```python
from build123d import *

# Parameters (mm, degrees)
EXTRUDE_1_DEPTH     = 10
SKETCH_2_W          = 80.6
SKETCH_2_H          = 36.6
CUT_EXTRUDE_1_DEPTH = 5
SKETCH_3_W          = 73
SKETCH_3_H          = 25
CUT_EXTRUDE_2_DEPTH = 115.512008104
CUT_EXTRUDE_3_DEPTH = 3
SKETCH_5_R          = 1.6
CUT_EXTRUDE_4_DEPTH = 112.950882087


with BuildPart() as part:
    # 草图1 → 凸台-拉伸1 (new body)
    with BuildSketch(Plane.XY):
        Polygon((0, 40), (0, 63), (-8, 63), (-8, 68), (5, 68), (5, 48.19405544), (13.19405544, 40), (70.80594456, 40), (79, 48.19405544), (79, 68), (92, 68), (92, 63), (84, 63), (84, 40), (84, 0), (0, 0), align=None)
    extrude(amount=EXTRUDE_1_DEPTH)

    # 草图2 → 切除-拉伸1 (cut)
    with BuildSketch(Plane.XY.offset(10)):
        with Locations((42, 20)):
            Rectangle(SKETCH_2_W, SKETCH_2_H)
    extrude(amount=-CUT_EXTRUDE_1_DEPTH, mode=Mode.SUBTRACT)

    # 草图3 → 切除-拉伸2 (cut, through all)
    with BuildSketch(Plane.XY.offset(5)):
        with Locations((42, 20)):
            Rectangle(SKETCH_3_W, SKETCH_3_H)
    extrude(amount=-CUT_EXTRUDE_2_DEPTH, mode=Mode.SUBTRACT)

    # 草图4 → 切除-拉伸3 (cut)
    with BuildSketch(Plane.XY.offset(5)):
        Polygon((77.017311929, 30.931067044), (82.3, 27.389990557), (82.3, 13.068303431), (77.017311929, 9.448536355), align=None)
        Polygon((6.982688071, 9.448536355), (6.982688071, 30.931067044), (1.7, 27.389990557), (1.7, 13.068303431), align=None)
    extrude(amount=-CUT_EXTRUDE_3_DEPTH, mode=Mode.SUBTRACT)

    # 草图5 → 切除-拉伸4 (cut, through all)
    with BuildSketch(Plane.XZ.offset(-63)):
        with Locations(Location((87.837450425, 4.830878187, 0), (0, 0, 270))):
            Circle(SKETCH_5_R)
        with Locations(Location((-3.837450425, 4.830878187, 0), (0, 0, 90))):
            Circle(SKETCH_5_R)
    extrude(amount=-CUT_EXTRUDE_4_DEPTH, mode=Mode.SUBTRACT)


solid = part.part
```
The listing builds one solid part. Answer for the finished solid, in the listing's coordinates (mm). A direction names the side the tool comes from. Give positions to 0.01 mm unless a question says otherwise; leave off trailing zeros. Write each loop counter-clockwise with the first axis right and the second up, starting at its lowest first coordinate (ties: lowest second). Pieces come first, ordered by that corner, then holes. Notation, with made-up numbers: (30, 30) - (87, 30) arc R12 cw to (87, 42) - close; hole circle Ø1 at (48.25, 78). An arc over 180 degrees is marked (long way). Use one line per item in the form item = value. Start each with the question number.
1) Find section B-B on x = 15. Determine the outline of the cut face in (y, z).
2) Flat-ended cylindrical pins translate along their axes: pin 1 Ø2.5 at (x, z) = (88, 6) entering from -Y; pin 2 Ø3 at (y, z) = (55, 7) entering from +X; pin 3 Ø2.5 at (x, z) = (-3.84, 4.83) entering from -Y; pin 4 Ø5 at (x, z) = (87.84, 4.83) entering from +Y. Find the tip coordinate at first contact, or state that the pin passes through.
3) The mould has two halves that part along Y. Classify faces 1 (the face through (85, 68, 5)), 2 (the face through (41, 5, 5)), 3 (the face through (79, 58, 5)): pulls with the +Y half, pulls with the -Y half, needs draft (parallel to the pull), parting line crosses it, or undercut.
4) Find section C-C on y = 36. Determine the outline of the cut face in (x, z), plus the area to 3 significant figures.
5) Consider line 1 along X through (y, z) = (58.5, 8.25); line 2 along X through (y, z) = (8, 3.75); line 3 along Y through (x, z) = (27, 4.5). Determine where each line is inside the solid, lowest interval first. Write a range as from..to.
6) A tool of negligible diameter and unlimited length cuts with its end or side. For faces 4 (the face through (78.5, 20, 1)), 5 (the face through (1.7, 20, 7)), 6 (the face through (84, 31, 5)), 7 (the face through (42, 40, 5)), from which of +Z, -Z, +X, -X, +Y, -Y can it reach the whole face along a straight path? Write none if from no direction.
7) Find section A-A on z = 8.5. Determine the outline of the cut face in (x, y).
Geometry results:
q1.outline = (0, 0) - (7.5, 0) - (7.5, 5) - (1.7, 5) - (1.7, 10) - (0, 10) - close; (32.5, 0) - (40, 0) - (40, 10) - (38.3, 10) - (38.3, 5) - (32.5, 5) - close
q2.pin_1 = 63
q2.pin_2 = 84
q2.pin_3 = through
q2.pin_4 = 68
q3.face_1 = pulls with the +Y half
q3.face_2 = undercut
q3.face_3 = needs draft
q4.outline = (0, 0) - (84, 0) - (84, 10) - (82.3, 10) - (82.3, 5) - (1.7, 5) - (1.7, 10) - (0, 10) - close
q4.area = 437 mm2
q5.line_1 = 0..5, 79..84
q5.line_2 = 0..5.5, 78.5..84
q5.line_3 = 0..7.5, 32.5..40
q6.face_4 = +Z, -Z
q6.face_5 = +Z
q6.face_6 = +Z, -Z, +X, -Y
q6.face_7 = +Z, -Z, +Y
q7.outline = (-8, 63) - (0, 63) - (0, 0) - (84, 0) - (84, 63) - (92, 63) - (92, 68) - (79, 68) - (79, 48.19) - (70.81, 40) - (13.19, 40) - (5, 48.19) - (5, 68) - (-8, 68) - close; hole (1.7, 1.7) - (82.3, 1.7) - (82.3, 38.3) - (1.7, 38.3) - close
